```python
from build123d import *
from build123d.topology import SkipClean

# Parameters (mm, degrees)
BOSS_EXTRUDE1_START     = 94
SKETCH1_R               = 21.9
SKETCH1_R_2             = 1.7
SKETCH1_R_3             = 6.4
BOSS_EXTRUDE1_DEPTH     = 3
BOSS_EXTRUDE2_START     = 91
BOSS_EXTRUDE2_DEPTH     = 27.5
BOSS_EXTRUDE3_START     = 45
BOSS_EXTRUDE3_DEPTH     = 18.5
BOSS_EXTRUDE7_START     = 94
BOSS_EXTRUDE7_DEPTH     = 49
CUT_EXTRUDE5_DEPTH      = 104.301419283
CUT_EXTRUDE5_DEPTH_BACK = 104.301419283
SKETCH4_W               = 8.985048174
SKETCH4_H               = 18
SKETCH4_R               = 2.25
CHAMFER3_SIZE           = 3
CHAMFER4_SIZE           = 1.5
FILLET2_R               = 2.5


with BuildPart() as part:
    # Sketch1 → Boss-Extrude1 (new body)
    with BuildSketch(Plane.XY.offset(BOSS_EXTRUDE1_START)):
        Circle(SKETCH1_R)
        with Locations((15.475, 0)):
            Circle(SKETCH1_R_2, mode=Mode.SUBTRACT)
        with Locations((7.7375, -13.401743124)):
            Circle(SKETCH1_R_2, mode=Mode.SUBTRACT)
        with Locations((-7.7375, -13.401743124)):
            Circle(SKETCH1_R_2, mode=Mode.SUBTRACT)
        with Locations((-15.475, 0)):
            Circle(SKETCH1_R_2, mode=Mode.SUBTRACT)
        with Locations((-7.7375, 13.401743124)):
            Circle(SKETCH1_R_2, mode=Mode.SUBTRACT)
        with Locations((7.7375, 13.401743124)):
            Circle(SKETCH1_R_2, mode=Mode.SUBTRACT)
        with Locations((0, -7)):
            Circle(SKETCH1_R_3, mode=Mode.SUBTRACT)
    extrude(amount=-BOSS_EXTRUDE1_DEPTH)

    # Sketch1<5> → Boss-Extrude2 (add)
    with BuildSketch(Plane.XY.offset(BOSS_EXTRUDE2_START)):
        with BuildLine():
            ThreePointArc((18.319661569, -12), (19.330787418, -10.292262036), (20.183161298, -8.5))
            Line((20.183161298, -8.5), (16.880758277, -8.5))
            ThreePointArc((16.880758277, -8.5), (0, -18.9), (-16.880758277, -8.5))
            Line((-16.880758277, -8.5), (-20.183161298, -8.5))
            ThreePointArc((-20.183161298, -8.5), (-19.330787418, -10.292262036), (-18.319661569, -12))
            ThreePointArc((-18.319661569, -12), (0, -21.9), (18.319661569, -12))
        make_face()
        with BuildLine():
            Line((-20.183161298, -8.5), (-16.880758277, -8.5))
            ThreePointArc((-16.880758277, -8.5), (-17.545632887, -7.025721786), (-18.082035284, -5.5))
            Line((-18.082035284, -5.5), (-21.198113124, -5.5))
            ThreePointArc((-21.198113124, -5.5), (-20.744938375, -7.018371022), (-20.183161298, -8.5))
        make_face()
        with BuildLine():
            Line((16.880758277, -8.5), (20.183161298, -8.5))
            ThreePointArc((20.183161298, -8.5), (20.744938375, -7.018371022), (21.198113124, -5.5))
            Line((21.198113124, -5.5), (18.082035284, -5.5))
            ThreePointArc((18.082035284, -5.5), (17.545632887, -7.025721786), (16.880758277, -8.5))
        make_face()
    extrude(amount=-BOSS_EXTRUDE2_DEPTH)

    # Sketch1<6> → Boss-Extrude3 (add)
    with SkipClean():  # the faces are left unmerged after this step: merging them gives an invalid solid
        with BuildSketch(Plane.XY.offset(BOSS_EXTRUDE3_START)):
            with BuildLine():
                Line((21.198113124, -5.5), (15.979987484, -5.5))
                ThreePointArc((15.979987484, -5.5), (0, -16.9), (-15.979987484, -5.5))
                Line((-15.979987484, -5.5), (-21.198113124, -5.5))
                ThreePointArc((-21.198113124, -5.5), (0, -21.9), (21.198113124, -5.5))
            make_face()
        extrude(amount=BOSS_EXTRUDE3_DEPTH)

    # Sketch1<11> → Boss-Extrude7 (add)
    with SkipClean():  # the faces are left unmerged after this step: merging them gives an invalid solid
        with BuildSketch(Plane.XY.offset(BOSS_EXTRUDE7_START)):
            with BuildLine():
                ThreePointArc((21.198113124, -5.5), (20.024388359, -8.867574124), (18.319661569, -12))
                Line((18.319661569, -12), (30.183161298, -12))
                Line((30.183161298, -12), (30.183161298, -8.5))
                Line((30.183161298, -8.5), (21.198113124, -8.5))
                Line((21.198113124, -8.5), (21.198113124, -5.5))
            make_face()
            with BuildLine():
                Line((-30.183161298, -12), (-18.319661569, -12))
                ThreePointArc((-18.319661569, -12), (-20.024388359, -8.867574124), (-21.198113124, -5.5))
                Line((-21.198113124, -5.5), (-21.198113124, -8.5))
                Line((-21.198113124, -8.5), (-30.183161298, -8.5))
                Line((-30.183161298, -8.5), (-30.183161298, -12))
            make_face()
        extrude(amount=-BOSS_EXTRUDE7_DEPTH)

    # Sketch4 → Cut-Extrude5 (cut, two sides: drawn at the far end of the back side and taken through both)
    with SkipClean():  # the faces are left unmerged after this step: merging them gives an invalid solid
        with BuildSketch(Plane(origin=(0, -8.5, 0), x_dir=(1, 0, 0), z_dir=(0, 1, 0)).offset(-CUT_EXTRUDE5_DEPTH_BACK)):
            with Locations((25.690637211, -70)):
                Rectangle(SKETCH4_W, SKETCH4_H)
            with Locations(Location((-25.690637211, -50, 0), (0, 0, 270))):
                Circle(SKETCH4_R)
            with Locations(Location((-25.690637211, -89, 0), (0, 0, 270))):
                Circle(SKETCH4_R)
            with Locations(Location((25.690637211, -86.5, 0), (0, 0, 270))):
                Circle(SKETCH4_R)
            with Locations(Location((25.690637211, -53.5, 0), (0, 0, 270))):
                Circle(SKETCH4_R)
        extrude(amount=CUT_EXTRUDE5_DEPTH + CUT_EXTRUDE5_DEPTH_BACK, mode=Mode.SUBTRACT)

    # Chamfer3
    # the kernel refuses this chamfer: 3 mm, written as the material it takes off along each edge
    with BuildSketch(Plane(origin=(0, 0, 63.5), x_dir=(0.9921367643584464, 0.1251584627915844, 0), z_dir=(-0.1251584627915844, 0.9921367643584464, 0))) as chamfer3_piece_1_section:
        Polygon((16.9 + CHAMFER3_SIZE, 0), (16.9, CHAMFER3_SIZE), (16.9, 0), align=None)
    chamfer3_piece_1 = revolve(axis=Axis((0, 0, 63.5), (0, 0, -1)), revolution_arc=194.379813793, mode=Mode.PRIVATE)
    chamfer3_piece_1 = chamfer3_piece_1 & Plane(origin=(0, 0, 61.502732277), x_dir=(0.8931618135876879, -0.4497354497354555, 0), z_dir=(0, 0, 1)) * Cylinder(18.9, 80, mode=Mode.PRIVATE)
    add(chamfer3_piece_1, mode=Mode.SUBTRACT)

    # Chamfer4
    chamfer4_edges = [part.edges().sort_by_distance(p)[0] for p in [
        (-6.4, -7, 91),
    ]]
    chamfer(chamfer4_edges, length=CHAMFER4_SIZE)

    # Fillet2
    fillet2_edges = [part.edges().sort_by_distance(p)[0] for p in [
        (21.198113124, -10.25, 79),
        (21.198113124, -10.25, 61),
        (30.183161298, -10.25, 61),
        (30.183161298, -10.25, 79),
        (-30.183161298, -10.25, 45),
        (-30.183161298, -10.25, 94),
        (30.183161298, -10.25, 45),
        (30.183161298, -10.25, 94),
    ]]
    fillet(fillet2_edges, radius=FILLET2_R)


solid = part.part
```
Build history of the part. All positions in model axes, mm. A direction names the side the tool comes from. Coordinates: 2 decimals unless noted, no trailing zeros. Order: outer loops, then holes, each group sorted by start corner. A loop starts at its lowest first (then second) coordinate and runs counter-clockwise, first axis right, second up. Notation, with made-up numbers: (88.5, 44.5) -> (103.5, 44.5) arc R16 cw to (103.5, 56.5) -> close; hole circle Ø1 at (78, 76). An arc over 180 degrees is marked (long way). Answer in a Markdown table with one row per item. Add a question column.
Q1. Band-saw the part on D-D, the plane y = 3.5. List the corners of the cut face in (x, z).
Q2. Which spindle directions (+Z, -Z, +X, -X, +Y, -Y) get a long thin tool onto all of the face, cutting with end or side? Do faces 4 (the face through (28, -8.5, 52)), 5 (the face through (26, -10, 61)), 6 (the face through (13.777, 0.075, 92.521)), 7 (the face through (-24, -12, 70)). Say none if no direction does.
Q3. Mould opens along X. For faces 1 (the face through (0, 2, 91)), 2 (the face through (20, -12, 70)), 3 (the face through (29.43, -10.23, 60.29)) say: +X half, -X half, draft (parallel to the pull), parting line (faces both ways), or undercut.
Q4. Band-saw the part on A-A, the plane x = 0. List the corners of the cut face in (y, z), then the cut area to 3 significant figures.
Q5. Band-saw the part on B-B, the plane z = 50. List the corners of the cut face in (x, y).
Q6. Drop flat-ended pins along their axis: pin 1 (4.5 mm diameter, centred on x = 25.5, z = 52, fed in from +Y); pin 2 (5 mm diameter, centred on x = 25.69, z = 53.5, fed in from -Y); pin 3 (2.5 mm diameter, centred on x = -18, z = 63, fed in from +Y). Give the stop position or say it passes through.
Q7. Band-saw the part on C-C, the plane z = 83.5. List the corners of the cut face in (x, y).
Q8. Wall check: line 1 along Y through (x, z) = (0, 74); line 2 along Z through (x, y) = (20, 0); line 3 along Y through (x, z) = (-24, 71). Give the ranges that are in metal, low to high. Write a range as [from, to].
Answers follow:
| question | item | result |
|---|---|---|
| 1 | outline | (-21.62, 91) -> (21.62, 91) -> (21.62, 94) -> (-21.62, 94) -> close |
| 2 | face 4 | +Z, -Z, +X, +Y |
| 2 | face 5 | +X, +Y, -Y |
| 2 | face 6 | +Z, -Z |
| 2 | face 7 | +Z, -Z, -X, -Y |
| 3 | face 1 | undercut |
| 3 | face 2 | draft |
| 3 | face 3 | +X half |
| 4 | outline | (-21.9, 45) -> (-16.9, 45) -> (-16.9, 60.5) -> (-18.9, 62.5) -> (-18.9, 91) -> (-14.9, 91) -> (-13.4, 92.5) -> (-13.4, 94) -> (-21.9, 94) -> close; (-0.6, 92.5) -> (0.9, 91) -> (21.9, 91) -> (21.9, 94) -> (-0.6, 94) -> close |
| 4 | area | 262 mm^2 |
| 5 | outline | (-30.18, -12) -> (-27.94, -12) -> (-27.94, -8.5) -> (-30.18, -8.5) -> close; (-23.44, -12) -> (-18.32, -12) arc R21.9 ccw to (18.32, -12) -> (30.18, -12) -> (30.18, -8.5) -> (21.2, -8.5) -> (21.2, -5.5) -> (15.98, -5.5) arc R16.9 cw to (-15.98, -5.5) -> (-21.2, -5.5) -> (-21.2, -8.5) -> (-23.44, -8.5) -> close |
| 6 | pin 1 | y = -8.5 |
| 6 | pin 2 | y = -12 |
| 6 | pin 3 | y = -5.5 |
| 7 | outline | (-30.18, -12) -> (-18.32, -12) arc R21.9 ccw to (18.32, -12) -> (30.18, -12) -> (30.18, -8.5) -> (21.2, -8.5) -> (21.2, -5.5) -> (18.08, -5.5) arc R18.9 cw to (-18.08, -5.5) -> (-21.2, -5.5) -> (-21.2, -8.5) -> (-30.18, -8.5) -> close |
| 8 | line 1 | [-21.9, -18.9] |
| 8 | line 2 | [91, 94] |
| 8 | line 3 | [-12, -8.5] |
